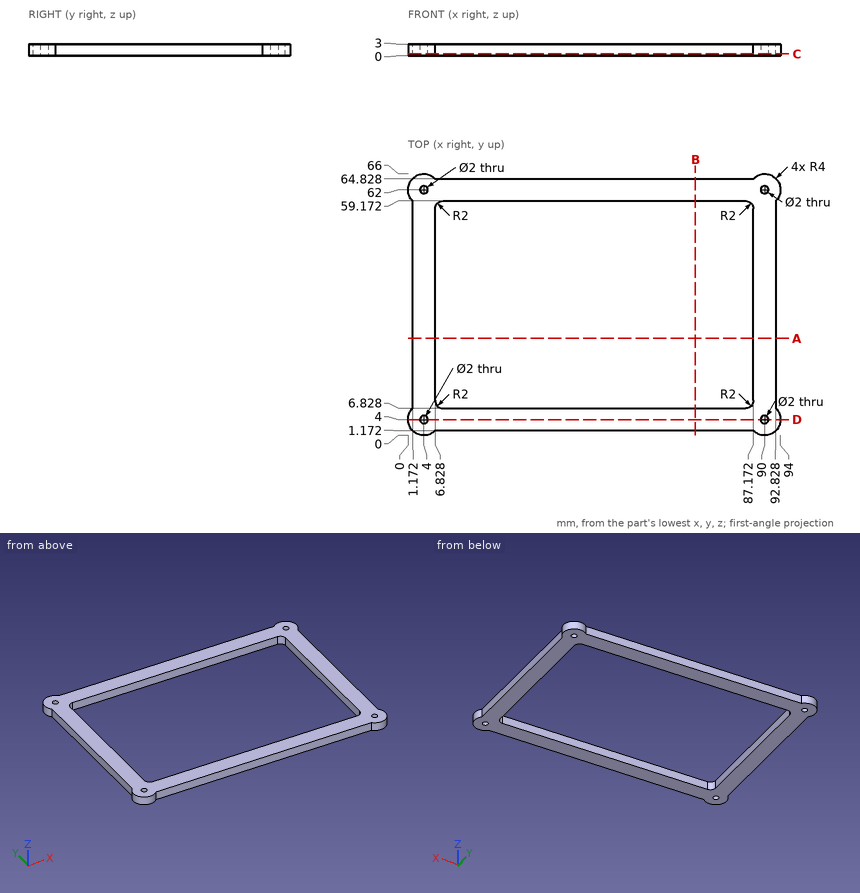
Geometry check sheet. Reference: drawing and pictorial views, mm from the part's lowest x, y, z. Round coordinates to 2 decimals unless told otherwise and drop trailing zeros. Loops run counter-clockwise (first coordinate to the right, second up) from the corner with the lowest first, then second, coordinate; pieces in that order, holes last. Notation, with made-up numbers: (-8, 73) - (27, 73) arc R20 ccw to (27, 102) - close; hole circle Ø5 at (17.25, 48.5). An arc over 180 degrees is marked (long way). Write item = value, one per line. Start each with the question number.
Q1. Section check B-B (x = 72.5). Record the boundary of the cut face in (y, z).
Q2. Section check D-D (y = 4). Record the boundary of the cut face in (x, z).
Q3. Depth check by flat-ended pin: P1, Ø2.5, axis at x = 4, y = 4, coming from the +Z side; P2, Ø12, axis at x = 26, y = 14.5, coming from the -Z side; P3, Ø1.5, axis at y = 24, z = 1, coming from the +X side; P4, Ø0.9, axis at x = 61.5, z = 2, coming from the +Y side. Enter the tip coordinate at first touch or a pass-through.
Q4. Section check C-C (z = 0.5). Record the boundary of the cut face in (x, y).
Q5. Thickness scan on L1, parallel to Y at x = 4, z = 1.6; L2, parallel to X at y = 52, z = 0.85; L3, parallel to Y at x = 16, z = 1.85. Record the ranges inside material, lowest first.
Q6. Section check A-A (y = 24.5). Record the boundary of the cut face in (x, z).
Derived:
q1.outline = (1.17, 0) - (6.83, 0) - (6.83, 3) - (1.17, 3) - close; (59.17, 0) - (64.83, 0) - (64.83, 3) - (59.17, 3) - close
q2.outline = (0, 0) - (3, 0) - (3, 3) - (0, 3) - close; (5, 0) - (89, 0) - (89, 3) - (5, 3) - close; (91, 0) - (94, 0) - (94, 3) - (91, 3) - close
q3.P1 = 3
q3.P2 = through
q3.P3 = 92.83
q3.P4 = 64.83
q4.outline = (1.17, 6.83) arc R4 ccw to (6.83, 1.17) - (87.17, 1.17) arc R4 ccw to (92.83, 6.83) - (92.83, 59.17) arc R4 ccw to (87.17, 64.83) - (6.83, 64.83) arc R4 ccw to (1.17, 59.17) - close; hole circle Ø2 at (4, 4); hole circle Ø2 at (4, 62); hole (6.83, 8.83) arc R2 ccw to (8.83, 6.83) - (85.17, 6.83) arc R2 ccw to (87.17, 8.83) - (87.17, 57.17) arc R2 ccw to (85.17, 59.17) - (8.83, 59.17) arc R2 ccw to (6.83, 57.17) - close; hole circle Ø2 at (90, 4); hole circle Ø2 at (90, 62)
q5.L1 = 0 to 3, 5 to 61, 63 to 66
q5.L2 = 1.17 to 6.83, 87.17 to 92.83
q5.L3 = 1.17 to 6.83, 59.17 to 64.83
q6.outline = (1.17, 0) - (6.83, 0) - (6.83, 3) - (1.17, 3) - close; (87.17, 0) - (92.83, 0) - (92.83, 3) - (87.17, 3) - close
